Read the model definition and answer for the solid it produces. Units are mm, in the model's axes. Face numbers are marked on the shaded views. Coordinates: 2 decimals unless noted, no trailing zeros. Write each loop counter-clockwise with the first axis right and the second up, starting at its lowest first coordinate (ties: lowest second). Pieces come first, ordered by that corner, then holes.
Item 1: Section D-D (x = 2) is taken. Give the vertices of the cut face in (y, z) (3 decimals).
Item 2: Section C-C (z = -31) is taken. Give the vertices of the cut face in (x, y), then the cut area to 3 significant figures.
Item 3: Straight lines are drawn through the part: probe 1 along X at (y, z) = (2.75, -16.5); probe 2 along Z at (x, y) = (-21, 7.25); probe 3 along Z at (x, y) = (27, 2.25). For each, find the intervals that lie inside material, in ascending order.
Item 4: Each of these flat-tipped pins is pushed along its axis until it touches: P1, Ø1.1, axis at x = 20.5, z = 38, coming from the +Y side; P2, Ø4, axis at x = 0, z = 43.5, coming from the +Y side (3 decimals); P3, Ø3, axis at x = 1.5, y = 5, coming from the +Z side. Where does it stop, or does it pass through?
Item 5: Section A-A (y = 5.25) is taken. Give the vertices of the cut face in (x, z), then the cut area to 3 significant figures.
Item 6: Determine the mould class of the marked faces 1 and 2 for opening direction X: released by +X, released by -X, zero draft, split by the parting line, or undercut.
Item 7: Section B-B (x = -10) is taken. Give the vertices of the cut face in (y, z).
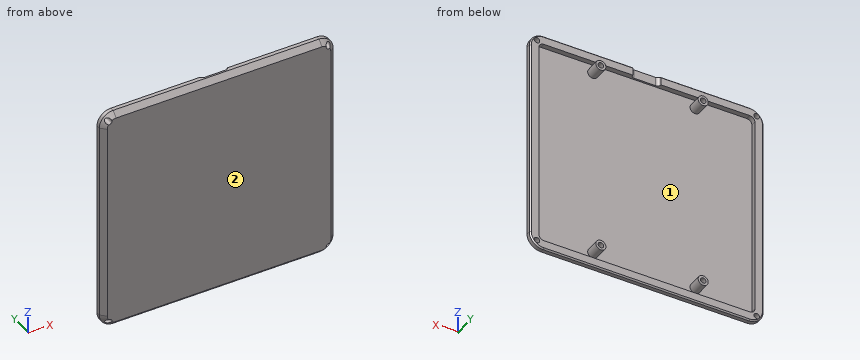
from build123d import *

# Parameters (mm, degrees)
BOSS_EXTRUDE1_DEPTH = 4
CUT_EXTRUDE1_DEPTH  = 2
CUT_EXTRUDE2_DEPTH  = 3.5
CHAMFER2_SIZE       = 2
CHAMFER3_SIZE       = 0.5
SKETCH4_R           = 2
SKETCH4_R_2         = 1.1
BOSS_EXTRUDE2_DEPTH = 5.5
SKETCH5_R           = 1.1
CUT_EXTRUDE3_DEPTH  = 4


with BuildPart() as part:
    # Sketch1 → Boss-Extrude1 (new body)
    with BuildSketch(Plane(origin=(0, 0, 0), x_dir=(1, 0, 0), z_dir=(0, 1, 0))):
        with BuildLine():
            Line((40.75, 45.000726786), (-40.75, 45.000726786))
            ThreePointArc((-40.75, 45.000726786), (-44.639601212, 43.389601212), (-46.250726786, 39.5))
            Line((-46.250726786, 39.5), (-46.250726786, -39.5))
            ThreePointArc((-46.250726786, -39.5), (-44.639601212, -43.389601212), (-40.75, -45.000726786))
            Line((-40.75, -45.000726786), (40.75, -45.000726786))
            ThreePointArc((40.75, -45.000726786), (44.639601212, -43.389601212), (46.250726786, -39.5))
            Line((46.250726786, -39.5), (46.250726786, 39.5))
            ThreePointArc((46.250726786, 39.5), (44.639601212, 43.389601212), (40.75, 45.000726786))
        make_face()
    extrude(amount=BOSS_EXTRUDE1_DEPTH)

    # Sketch2 → Cut-Extrude1 (cut)
    with BuildSketch(Plane(origin=(0, 4, 0), x_dir=(1, 0, 0), z_dir=(0, 1, 0))):
        with BuildLine():
            Line((-42.750726786, 39.5), (-42.750726786, -39.5))
            ThreePointArc((-42.750726786, -39.5), (-42.164727477, -40.914727477), (-40.75, -41.500726786))
            Line((-40.75, -41.500726786), (40.75, -41.500726786))
            ThreePointArc((40.75, -41.500726786), (42.164727477, -40.914727477), (42.750726786, -39.5))
            Line((42.750726786, -39.5), (42.750726786, 39.5))
            ThreePointArc((42.750726786, 39.5), (42.164727477, 40.914727477), (40.75, 41.500726786))
            Line((40.75, 41.500726786), (-40.75, 41.500726786))
            ThreePointArc((-40.75, 41.500726786), (-42.164727477, 40.914727477), (-42.750726786, 39.5))
        make_face()
    extrude(amount=-CUT_EXTRUDE1_DEPTH, mode=Mode.SUBTRACT)

    # Sketch3 → Cut-Extrude2 (cut)
    with BuildSketch(Plane.XY.offset(45.000726786)):
        with BuildLine():
            Line((-4.25, 5.325), (4.25, 5.325))
            ThreePointArc((4.25, 5.325), (5.575, 4), (4.25, 2.675))
            Line((4.25, 2.675), (-4.25, 2.675))
            ThreePointArc((-4.25, 2.675), (-5.575, 4), (-4.25, 5.325))
        make_face()
    extrude(amount=-CUT_EXTRUDE2_DEPTH, mode=Mode.SUBTRACT)

    # Chamfer2
    chamfer2_edges = [part.edges().sort_by_distance(p)[0] for p in [
        (44.639601212, 0, -43.389601212),
        (46.250726786, 0, 0),
        (44.639601212, 0, 43.389601212),
        (0, 0, 45.000726786),
        (-44.639601212, 0, 43.389601212),
        (-46.250726786, 0, 0),
        (-44.639601212, 0, -43.389601212),
        (0, 0, -45.000726786),
    ]]
    chamfer(chamfer2_edges, length=CHAMFER2_SIZE)

    # Chamfer3
    chamfer3_edges = [part.edges().sort_by_distance(p)[0] for p in [
        (46.250726786, 4, 0),
        (44.639601212, 4, -43.389601212),
        (0, 4, -45.000726786),
        (-44.639601212, 4, -43.389601212),
        (-46.250726786, 4, 0),
        (-44.639601212, 4, 43.389601212),
        (-23.1625, 4, 45.000726786),
        (23.1625, 4, 45.000726786),
        (44.639601212, 4, 43.389601212),
    ]]
    chamfer(chamfer3_edges, length=CHAMFER3_SIZE)

    # Sketch4 → Boss-Extrude2 (add)
    with BuildSketch(Plane(origin=(0, 2, 0), x_dir=(1, 0, 0), z_dir=(0, 1, 0))):
        with Locations((-20.250726786, -38.000726786)):
            Circle(SKETCH4_R)
        with Locations((-20.250726786, -38.000726786)):
            Circle(SKETCH4_R_2, mode=Mode.SUBTRACT)
        with Locations((20.250726786, -38.000726786)):
            Circle(SKETCH4_R)
        with Locations((20.250726786, -38.000726786)):
            Circle(SKETCH4_R_2, mode=Mode.SUBTRACT)
        with Locations((20.250726786, 38.000726786)):
            Circle(SKETCH4_R)
        with Locations((20.250726786, 38.000726786)):
            Circle(SKETCH4_R_2, mode=Mode.SUBTRACT)
        with Locations((-20.250726786, 38.000726786)):
            Circle(SKETCH4_R)
        with Locations((-20.250726786, 38.000726786)):
            Circle(SKETCH4_R_2, mode=Mode.SUBTRACT)
    extrude(amount=BOSS_EXTRUDE2_DEPTH)

    # Sketch5 → Cut-Extrude3 (cut)
    with BuildSketch(Plane.XZ):
        with Locations((-43.500363393, 42.250363393)):
            Circle(SKETCH5_R)
        with Locations((43.500363393, 42.250363393)):
            Circle(SKETCH5_R)
        with Locations((43.500363393, -42.250363393)):
            Circle(SKETCH5_R)
        with Locations((-43.500363393, -42.250363393)):
            Circle(SKETCH5_R)
    extrude(amount=-CUT_EXTRUDE3_DEPTH, mode=Mode.SUBTRACT)


solid = part.part
Established:
1. outline: (0, -43.001) - (2, -45.001) - (3.5, -45.001) - (4, -44.501) - (4, -41.501) - (2, -41.501) - (2, 41.501) - (2.675, 41.501) - (2.675, 45.001) - (2, 45.001) - (0, 43.001) - close
2. outline: (-46.25, 2) - (-44.25, 0) - (44.25, 0) - (46.25, 2) - (46.25, 3.5) - (45.75, 4) - (42.75, 4) - (42.75, 2) - (-42.75, 2) - (-42.75, 4) - (-45.75, 4) - (-46.25, 3.5) - close
2. area: 195 mm2
3. probe 1: x = -46.25 to -42.75, 42.75 to 46.25
3. probe 2: z = -39.86 to -38.81, -37.2 to -36.15, 36.15 to 37.2, 38.81 to 39.86
3. probe 3: z = -45 to -41.5, 41.5 to 45
4. P1: stops at y = 2
4. P2: stops at y = 2.675
4. P3: stops at z = -41.5
5. outline: circle Ø4 at (-20.25, -38); circle Ø4 at (-20.25, 38); circle Ø4 at (20.25, -38); circle Ø4 at (20.25, 38); hole circle Ø2.2 at (-20.25, -38); hole circle Ø2.2 at (-20.25, 38); hole circle Ø2.2 at (20.25, -38); hole circle Ø2.2 at (20.25, 38)
5. area: 35.1 mm2
6. face 1: undercut
6. face 2: zero draft
7. outline: (0, -43) - (2, -45) - (3.5, -45) - (4, -44.5) - (4, -41.5) - (2, -41.5) - (2, 41.5) - (4, 41.5) - (4, 44.5) - (3.5, 45) - (2, 45) - (0, 43) - close
